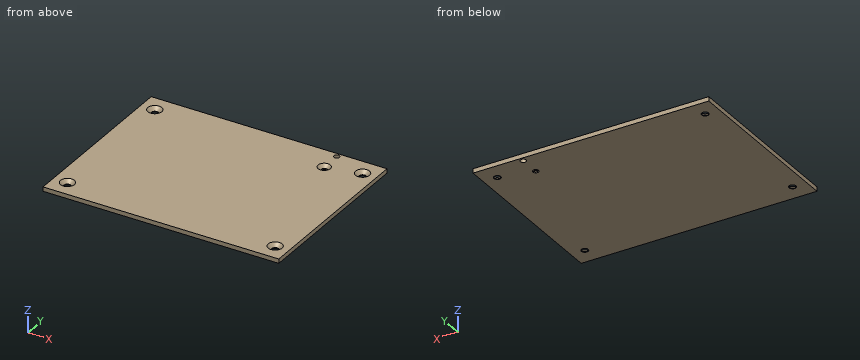
from build123d import *

# Parameters (mm, degrees)
SKETCH1_W                                    = 109.5
SKETCH1_H                                    = 83
BOSS_EXTRUDE1_DEPTH                          = 2
CSK_FOR_M3_FLAT_COUNTERSUNK_HEAD_SCR_2_COUNT = 2
CSK_FOR_M3_FLAT_COUNTERSUNK_HEAD_SCR_2_PITCH = 67
CSK_FOR_M3_FLAT_COUNTERSUNK_HEAD_SCR_3_COUNT = 2
CSK_FOR_M3_FLAT_COUNTERSUNK_HEAD_SCR_3_PITCH = 117.478721478
CSK_FOR_M3_FLAT_COUNTERSUNK_HEAD_SCR_4_COUNT = 2
CSK_FOR_M3_FLAT_COUNTERSUNK_HEAD_SCR_4_PITCH = 96.5
F_2_6_2_6_DIAMETER_HOLE1_D                   = 2.6


with BuildPart() as part:
    # Sketch1 → Boss-Extrude1 (new body)
    with BuildSketch(Plane.XY):
        with Locations((0, -41.5)):
            Rectangle(SKETCH1_W, SKETCH1_H)
    extrude(amount=BOSS_EXTRUDE1_DEPTH)

    # Sketch3 → CSK for M3 Flat Countersunk Head Screw1 (revolve, cut)
    with BuildSketch(Plane(origin=(-48.25, -8, 2), x_dir=(0, -1, 0), z_dir=(1, 0, 0))):
        Polygon((0, 0), (0, 2), (1.6, 2), (1.6, 1.65), (3.25, 0), align=None)
    csk_for_m3_flat_countersunk_head_screw1 = revolve(axis=Axis((-48.25, -8, 8.35), (0, 0, -1)), mode=Mode.SUBTRACT)

    # CSK for M3 Flat Countersunk Head Scr 2: CSK for M3 Flat Countersunk Head Screw1 ×2
    with Locations(*[(0, -i * CSK_FOR_M3_FLAT_COUNTERSUNK_HEAD_SCR_2_PITCH, 0) for i in range(1, CSK_FOR_M3_FLAT_COUNTERSUNK_HEAD_SCR_2_COUNT)]):
        add(csk_for_m3_flat_countersunk_head_screw1, mode=Mode.SUBTRACT)

    # CSK for M3 Flat Countersunk Head Scr 3: CSK for M3 Flat Countersunk Head Screw1 ×2
    with Locations(*[Vector(0.8214253507895062, -0.570316046662144, 0) * (i * CSK_FOR_M3_FLAT_COUNTERSUNK_HEAD_SCR_3_PITCH) for i in range(1, CSK_FOR_M3_FLAT_COUNTERSUNK_HEAD_SCR_3_COUNT)]):
        add(csk_for_m3_flat_countersunk_head_screw1, mode=Mode.SUBTRACT)

    # CSK for M3 Flat Countersunk Head Scr 4: CSK for M3 Flat Countersunk Head Screw1 ×2
    with Locations(*[(i * CSK_FOR_M3_FLAT_COUNTERSUNK_HEAD_SCR_4_PITCH, 0, 0) for i in range(1, CSK_FOR_M3_FLAT_COUNTERSUNK_HEAD_SCR_4_COUNT)]):
        add(csk_for_m3_flat_countersunk_head_screw1, mode=Mode.SUBTRACT)

    # Sketch5 → CSK for M2.5 Flat Countersunk Head Screw1 (revolve, cut)
    with BuildSketch(Plane(origin=(32.65, -11.6, 2), x_dir=(0, -1, 0), z_dir=(1, 0, 0))):
        Polygon((0, 0), (0, 2), (1.35, 2), (1.35, 1.5), (2.85, 0), align=None)
    revolve(axis=Axis((32.65, -11.6, 8.35), (0, 0, -1)), mode=Mode.SUBTRACT)

    # Ø2.6 (2.6) Diameter Hole1 (through all)
    with Locations(Plane.XY.offset(2)):
        with Locations((32.65, -2.07)):
            Hole(F_2_6_2_6_DIAMETER_HOLE1_D / 2)


solid = part.part
Verification items for the finished model (mm, model axes). Give positions to 0.01 mm unless a question says otherwise; leave off trailing zeros. Write each loop counter-clockwise with the first axis right and the second up, starting at its lowest first coordinate (ties: lowest second). Pieces come first, ordered by that corner, then holes.
(1) Cross-section at A-A (x = 48.25). Enter the section's corners in (y, z).
(2) Cross-section at C-C (y = -2.07). Enter the section's corners in (x, z), plus the area to 3 significant figures.
(3) Gauge pin test, flat ends, axial feed: pin 1 (3.5 mm diameter, centred on x = -48.25, y = -8, fed in from +Z); pin 2 (2.5 mm diameter, centred on x = 32.65, y = -11.6, fed in from +Z). Record the tip position at first contact, or that the pin passes through.
(4) Cross-section at B-B (y = -75). Enter the section's corners in (x, z).
(5) Material ranges on line 1 (Y direction, x = -48.25, z = 0.15); line 2 (X direction, y = -75, z = 0.25); line 3 (X direction, y = -10, z = 1.6), recorded low to high.
Worked out:
1. outline: (-83, 0) - (-76.6, 0) - (-76.6, 0.35) - (-78.25, 2) - (-83, 2) - close; (-73.4, 0) - (-9.6, 0) - (-9.6, 0.35) - (-11.25, 2) - (-71.75, 2) - (-73.4, 0.35) - close; (-6.4, 0) - (0, 0) - (0, 2) - (-4.75, 2) - (-6.4, 0.35) - close
2. outline: (-54.75, 0) - (31.35, 0) - (31.35, 2) - (-54.75, 2) - close; (33.95, 0) - (54.75, 0) - (54.75, 2) - (33.95, 2) - close
2. area: 214 mm2
3. pin 1: stops at z = 0.5
3. pin 2: passes through
4. outline: (-54.75, 0) - (-49.85, 0) - (-49.85, 0.35) - (-51.5, 2) - (-54.75, 2) - close; (-46.65, 0) - (46.65, 0) - (46.65, 0.35) - (45, 2) - (-45, 2) - (-46.65, 0.35) - close; (49.85, 0) - (54.75, 0) - (54.75, 2) - (51.5, 2) - (49.85, 0.35) - close
5. line 1: y = -83 to -76.6, -73.4 to -9.6, -6.4 to 0
5. line 2: x = -54.75 to -49.85, -46.65 to 46.65, 49.85 to 54.75
5. line 3: x = -54.75 to -50.28, -46.22 to 30.79, 34.51 to 46.22, 50.28 to 54.75
